Source: CAD feature listing. Evaluate the final solid. Frame: model axes, mm. A direction names the side the tool comes from. Give positions to 0.01 mm unless a question says otherwise; leave off trailing zeros. Loops run counter-clockwise (first coordinate to the right, second up) from the corner with the lowest first, then second, coordinate; pieces in that order, holes last. Notation, with made-up numbers: (25, -4.5) - (58, -4.5) arc R6 cw to (58, 0.5) - close; hole circle Ø4 at (40.25, -31). An arc over 180 degrees is marked (long way). Put each result on its own line as item: value.
```python
from build123d import *

# Parameters (mm, degrees)
SKETCH_1_W          = 51.5
SKETCH_1_H          = 34.15
SKETCH_1_W_2        = 31.5
SKETCH_1_H_2        = 14.15
EXTRUDE_1_DEPTH     = 12.25
SKETCH_2_R          = 1.91
CUT_EXTRUDE_1_DEPTH = 34.236736076
SKETCH_4_W          = 13
SKETCH_4_H          = 13.91
EXTRUDE_1_2_DEPTH   = 74.82
SKETCH_5_W          = 13.91
SKETCH_5_H          = 16.23
EXTRUDE_2_DEPTH     = 16
SKETCH_7_R          = 25.25
SKETCH_7_R_2        = 15.25
EXTRUDE_2_2_DEPTH   = 16.23
SKETCH_15_R         = 1.91
CUT_EXTRUDE_6_DEPTH = 97.964478439
SKETCH_16_W         = 13.91
SKETCH_16_H         = 16.23
EXTRUDE_4_DEPTH     = 10
SKETCH_17_R         = 1.91
CUT_EXTRUDE_7_DEPTH = 102.16913771


with BuildPart() as part:
    # Sketch 1 → Extrude 1 (new body)
    with BuildSketch(Plane(origin=(0, 0, 0), x_dir=(1, 0, 0), z_dir=(0, 1, 0))):
        Rectangle(SKETCH_1_W, SKETCH_1_H)
        Rectangle(SKETCH_1_W_2, SKETCH_1_H_2, mode=Mode.SUBTRACT)
    extrude(amount=EXTRUDE_1_DEPTH)

    # Sketch 2 → Cut-Extrude 1 (cut, through all)
    with BuildSketch(Plane(origin=(0, 12.25, 0), x_dir=(1, 0, 0), z_dir=(0, 1, 0))):
        with Locations(Location((-20.75, 0, 0), (0, 0, 270))):
            Circle(SKETCH_2_R)
        with Locations(Location((20.75, 0, 0), (0, 0, 270))):
            Circle(SKETCH_2_R)
    extrude(amount=-CUT_EXTRUDE_1_DEPTH, mode=Mode.SUBTRACT)

    # Sketch 4 → Extrude 1 2 (add)
    with BuildSketch(Plane.XZ):
        with Locations((19.25, 0)):
            Rectangle(SKETCH_4_W, SKETCH_4_H)
    extrude(amount=EXTRUDE_1_2_DEPTH)

    # Sketch 5 → Extrude 2 (add)
    with BuildSketch(Plane.ZY.offset(-12.75)):
        with Locations((0, -66.705)):
            Rectangle(SKETCH_5_W, SKETCH_5_H)
    extrude(amount=EXTRUDE_2_DEPTH)

    # Sketch 7 → Extrude 2 2 (add)
    with BuildSketch(Plane(origin=(3.626674765, -74.82, 0), x_dir=(1, 0, 0), z_dir=(0, -1, 0))):
        with Locations((-30.978154344, 0)):
            Circle(SKETCH_7_R)
        with Locations((-30.978154344, 0)):
            Circle(SKETCH_7_R_2, mode=Mode.SUBTRACT)
    extrude(amount=-EXTRUDE_2_2_DEPTH)

    # Sketch 15 → Cut-Extrude 6 (cut, through all)
    with BuildSketch(Plane(origin=(0, 0, -6.955), x_dir=(-1, 0, 0), z_dir=(0, 0, -1))):
        with Locations((-4.835883248, -66.705)):
            Circle(SKETCH_15_R)
    extrude(amount=-CUT_EXTRUDE_6_DEPTH, mode=Mode.SUBTRACT)

    # Sketch 16 → Extrude 4 (add)
    with BuildSketch(Plane(origin=(-60, 0, 0), x_dir=(0, 0, -1), z_dir=(1, 0, 0))):
        with Locations((0, -66.705)):
            Rectangle(SKETCH_16_W, SKETCH_16_H)
    extrude(amount=EXTRUDE_4_DEPTH)

    # Sketch 17 → Cut-Extrude 7 (cut, through all)
    with BuildSketch(Plane(origin=(0, 0, -6.955), x_dir=(-1, 0, 0), z_dir=(0, 0, -1))):
        with Locations((55.812362827, -66.705)):
            Circle(SKETCH_17_R)
    extrude(amount=-CUT_EXTRUDE_7_DEPTH, mode=Mode.SUBTRACT)


solid = part.part
```
1) Pin query (flat end, axial travel): P1, Ø5, axis at x = -55.81, y = -66.7, coming from the -Z side (3 decimals); P2, Ø4.5, axis at x = 4.84, y = -66.7, coming from the +Z side (3 decimals); P3, Ø12, axis at x = 7, z = 15, coming from the -Y side. Return the tip coordinate at first contact, or that it passes through.
Check result:
P1: z = -6.955
P2: z = 6.955
P3: y = 0
2) Material intervals for line 1 along X through (y, z) = (4, 0); line 2 along Z through (x, y) = (12.5, 7) (3 decimals); line 3 along Y through (x, z) = (-13.5, -8), sorted ascending. Write a range as [from, to].
Check result:
line 1: [-25.75, -22.66], [-18.84, -15.75], [15.75, 18.84], [22.66, 25.75]
line 2: [-17.075, -7.075], [7.075, 17.075]
line 3: [-74.82, -58.59], [0, 12.25]
3) Access query for faces 4 (the cylindrical face through (-27.808, -66.819, -25.246)), 5 (the flat face through (14, 0, 0)), 6 (the flat face through (-15.75, 6, 0)). Directions: +Z, -Z, +X, -X, +Y, -Y. A direction counts if a zero-diameter tool reaches every point of the face in a straight line with its end or side. Return the directions, or none.
Check result:
face 4: -Z, -Y
face 5: +Y
face 6: +Y, -Y
4) Mould query, pull axis X, two halves, no side actions, for faces 1 (the flat face through (21, 0, 0)), 2 (the flat face through (-25.75, 6, 0)), 3 (the flat face through (0, 6, -17.075)). Classes: pulls with the +X half, pulls with the -X half, needs draft (parallel to the pull), parting line crosses it, or undercut.
Check result:
face 1: undercut
face 2: pulls with the -X half
face 3: needs draft
5) Section query A-A, the plane z = 0. Output: boundary loops of the cut face in (x, y) (3 decimals), plus the area to 3 significant figures.
Check result:
outline: (-60, -74.82) - (-42.601, -74.82) - (-42.601, -58.59) - (-60, -58.59) - close; (-25.75, 0) - (-22.66, 0) - (-22.66, 12.25) - (-25.75, 12.25) - close; (-18.84, 0) - (-15.75, 0) - (-15.75, 12.25) - (-18.84, 12.25) - close; (-12.101, -74.82) - (25.75, -74.82) - (25.75, 12.25) - (22.66, 12.25) - (22.66, 0) - (18.84, 0) - (18.84, 12.25) - (15.75, 12.25) - (15.75, 0) - (12.75, 0) - (12.75, -58.59) - (-12.101, -58.59) - close; hole circle Ø3.82 at (-55.812, -66.705); hole circle Ø3.82 at (4.836, -66.705)
area: 1,790 mm²
6) Section query C-C, the plane x = 20.75. Output: boundary loops of the cut face in (y, z) (3 decimals), plus the area to 3 significant figures.
Check result:
outline: (-74.82, -6.955) - (0, -6.955) - (0, -17.075) - (12.25, -17.075) - (12.25, -1.91) - (0, -1.91) - (0, 1.91) - (12.25, 1.91) - (12.25, 17.075) - (0, 17.075) - (0, 6.955) - (-74.82, 6.955) - close
area: 1,410 mm²
7) Section query D-D, the plane x = -20.75. Output: boundary loops of the cut face in (y, z) (3 decimals), plus the area to 3 significant figures.
Check result:
outline: (-74.82, -24.372) - (-58.59, -24.372) - (-58.59, -13.747) - (-74.82, -13.747) - close; (-74.82, 13.747) - (-58.59, 13.747) - (-58.59, 24.372) - (-74.82, 24.372) - close; (0, -17.075) - (12.25, -17.075) - (12.25, -1.91) - (0, -1.91) - close; (0, 1.91) - (12.25, 1.91) - (12.25, 17.075) - (0, 17.075) - close
area: 716 mm²
8) Section query B-B, the plane y = -60. Output: boundary loops of the cut face in (x, z) (3 decimals), plus the area to 3 significant figures.
Check result:
outline: (-60, -6.955) - (-51.625, -6.955) arc R25.25 ccw to (-3.078, -6.955) - (25.75, -6.955) - (25.75, 6.955) - (-3.078, 6.955) arc R25.25 ccw to (-51.625, 6.955) - (-60, 6.955) - close; hole circle Ø30.5 at (-27.351, 0)
area: 1,770 mm²
